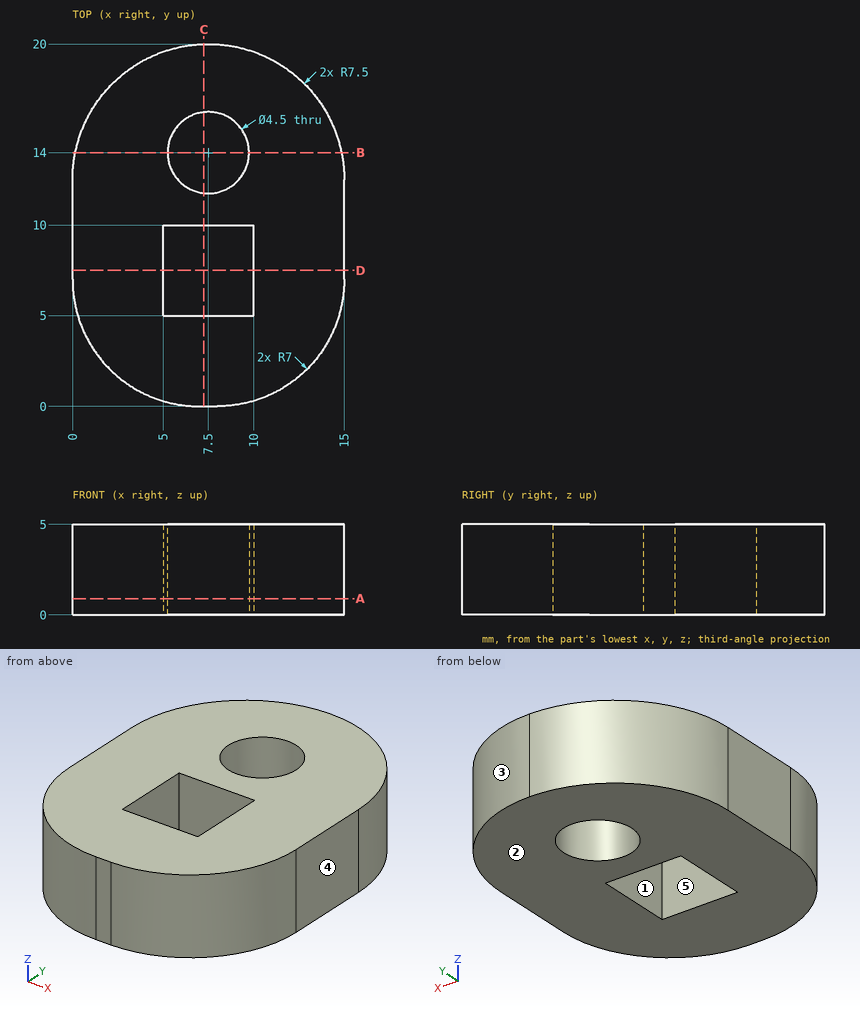
Answer from the drawing. Dimensions are ordinates in mm from the lowest x, y and z of the part. A direction names the side the tool comes from. Give positions to 0.01 mm unless a question says otherwise; leave off trailing zeros. Order: outer loops, then holes, each group sorted by start corner. A loop starts at its lowest first (then second) coordinate and runs counter-clockwise, first axis right, second up.
Item 1: For a pull along Y with two mould halves and no side action, classify the marked faces 1, 2 and 3 as pulls with the +Y half, pulls with the -Y half, needs draft (parallel to the pull), parting line crosses it, or undercut.
From the geometry:
face 1: undercut
face 2: needs draft
face 3: pulls with the +Y half
Item 2: The part is cut by section D-D, the plane y = 7.5. Give the vertices of the cut face in (x, z), and give its area (3 significant figures).
From the geometry:
outline: (0, 0) - (5, 0) - (5, 5) - (0, 5) - close; (10, 0) - (15, 0) - (15, 5) - (10, 5) - close
area: 50.0 mm2
Item 3: The part is cut by section A-A, the plane z = 0.9. Count the separate pieces of the cut face and the enclosed holes in it, and give its area (3 significant figures).
From the geometry:
separate pieces: 1
enclosed holes: 2
area: 214 mm2
Item 4: The part is cut by section B-B, the plane y = 14. Give the vertices of the cut face in (x, z), and give its area (3 significant figures).
From the geometry:
outline: (0.15, 0) - (5.25, 0) - (5.25, 5) - (0.15, 5) - close; (9.75, 0) - (14.85, 0) - (14.85, 5) - (9.75, 5) - close
area: 51.0 mm2
Item 5: Given pin 1 Ø1.5 at (y, z) = (13.5, 3.5) entering from -X; pin 2 Ø2 at (y, z) = (3.5, 1) entering from -X; pin 3 Ø1 at (x, z) = (9, 3.5) entering from -Y, each flat-ended and moving along its own axis, determine where each tip first touches the part or whether it passes through.
From the geometry:
pin 1: stops at x = 0
pin 2: stops at x = 0.46
pin 3: stops at y = 0.02
Item 6: Which of the six approach directions +Z, -Z, +X, -X, +Y, -Y give full straight-line access (tool end or side, diameter ignored) to the marked faces 4 and 5?
From the geometry:
face 4: +Z, -Z, +X, +Y, -Y
face 5: +Z, -Z
Item 7: The part is cut by section C-C, the plane x = 7.25. Give the vertices of the cut face in (y, z), and give its area (3 significant figures).
From the geometry:
outline: (0, 0) - (5, 0) - (5, 5) - (0, 5) - close; (10, 0) - (11.76, 0) - (11.76, 5) - (10, 5) - close; (16.24, 0) - (20, 0) - (20, 5) - (16.24, 5) - close
area: 52.6 mm2
Item 8: Find the intervals of material crossed by probe 1 along Y at (x, z) = (7.5, 3.2); probe 2 along Y at (x, z) = (8.5, 0.2); probe 3 along X at (y, z) = (6.25, 2.1), in increasing order.
From the geometry:
probe 1: y = 0 to 5, 10 to 11.75, 16.25 to 20
probe 2: y = 0.02 to 5, 10 to 11.98, 16.02 to 19.93
probe 3: x = 0.04 to 5, 10 to 14.96
